Could you check a few things on this model? Use its own coordinates, in mm. A direction names the side the tool comes from. Round coordinates to 2 decimals unless told otherwise and drop trailing zeros. Order: outer loops, then holes, each group sorted by start corner. A loop starts at its lowest first (then second) coordinate and runs counter-clockwise, first axis right, second up.
```python
from build123d import *

# Parameters (mm, degrees)
F1_DEPTH  = 3
F3_DEPTH  = 10
F5_DEPTH  = 25
F6_W      = 4.4599839021
F6_H      = 15.0388356149
F6_W_2    = 4
F7_DEPTH  = 3
F8_R      = 1.5
F9_DEPTH  = 25
F11_DEPTH = 25


with BuildPart() as f1:
    # F0 (on Top) → F1 (new body)
    with BuildSketch(Plane.XY):
        with BuildLine():
            Line((1.9915475706, -41), (1.9915475706, -25.9236135266))
            ThreePointArc((1.9915475706, -25.9236135266), (0.0084775482, 25.9999986179), (-2.0084524294, -25.9223092883))
            Line((-2.0084524294, -25.9223092883), (-2.0084524294, -41))
            Line((-2.0084524294, -41), (1.9915475706, -41))
        make_face()
    extrude(amount=-F1_DEPTH)

    # F2 (on face) → F3 (join)
    with BuildSketch(Plane.XY):
        with BuildLine():
            Line((1.9915475706, 0), (-2.0153727382, 0))
            Line((-2.0153727382, 0), (-2.0153727382, -25.9217721756))
            ThreePointArc((-2.0153727382, -25.9217721756), (-2.0119126018, -25.9220409629), (-2.0084524294, -25.9223092883))
            Line((-2.0084524294, -25.9223092883), (-2.0084524294, -41))
            Line((-2.0084524294, -41), (1.9915475706, -41))
            Line((1.9915475706, -41), (1.9915475706, -25.9236135266))
            Line((1.9915475706, -25.9236135266), (1.9915475706, 0))
        make_face()
    extrude(amount=F3_DEPTH)

    # F4 (on face) → F5 (cut)
    with BuildSketch(Plane.YZ.offset(1.9915475706)):
        Polygon((-29.4827464968, 10), (0, 0), (0, 10), align=None)
    extrude(amount=-F5_DEPTH, mode=Mode.SUBTRACT)

    # F6 (on face) → F7 (cut)
    with BuildSketch(Plane(origin=(0, 0, -3), x_dir=(1, 0, 0), z_dir=(0, 0, -1))):
        with Locations((-0.0513555715, 33.4805821925)):
            Rectangle(F6_W, F6_H)
        with Locations((-0.0084524294, 33.4805821925)):
            Rectangle(F6_W_2, F6_H)
    extrude(amount=-F7_DEPTH, mode=Mode.SUBTRACT)

    # F8 (on face) → F9 (cut)
    with BuildSketch(Plane.YZ.offset(1.9915475706)):
        with Locations((-36, 5)):
            Circle(F8_R)
    extrude(amount=-F9_DEPTH, mode=Mode.SUBTRACT)

    # F10 (on face) → F11 (cut)
    with BuildSketch(Plane.YZ.offset(1.9915475706)):
        Polygon((-25.9236135266, -3), (-25.9236135266, 0), (-41, 1.5707125422), (-41, 0), (-25.9611643851, 0), (-25.9611643851, -3), align=None)
    extrude(amount=-F11_DEPTH, mode=Mode.SUBTRACT)


solid = f1.part
```
Q1. Imagine slicing it at C-C, the plane y = -36. Please give me the cut outline in (x, z), then the cut area to 3 significant figures.
Q2. For faces 4 (the flat face through (-2.015, -19, 2)), 5 (the flat face through (0, -41, 6)), 6 (the flat face through (0, -25.924, -2)), which set-ups out of +Z, -Z, +X, -X, +Y, -Y let a thin tool reach every point of the face, with its end or its side?
Q3. Imagine slicing it at D-D, the plane y = -19. Please give me the cut outline in (x, z), then the cut area to 3 significant figures.
Q4. We'd pull the mould along Z, two halves only. Please class faces 1 (the cylindrical face through (0, -37.2, 4.1)), 2 (the flat face through (0.02, -33.356, 0.774)), 3 (the flat face through (1.992, -25, 4)): released by +Z, released by -Z, zero draft, split by the parting line, or undercut.
Q5. For P1, Ø4.5, axis at y = -17.5, z = 3.5, coming from the -X side; P2, Ø6, axis at y = -9, z = 5, coming from the +X side; P3, Ø5, axis at x = -18.5, z = 1.5, coming from the -Y side; P4, Ø3, axis at x = 14.5, z = 3, coming from the +Y side, each with a flat end and sliding along its axis, tell me the tip position at first contact or that it passes through.
Q6. I need wall thicknesses on L1, parallel to Z at x = -1, y = -36; L2, parallel to Z at x = 23, y = -5.5; L3, parallel to X at y = -7, z = 2. Which ranges of each line are inside material? Lowest first, please.
Q7. Imagine slicing it at A-A, the plane x = 0. Please give me the cut outline in (y, z).
Filled in:
1. outline: (-2.01, 1.05) - (1.99, 1.05) - (1.99, 3.5) - (-2.01, 3.5) - close; (-2.01, 6.5) - (1.99, 6.5) - (1.99, 10) - (-2.01, 10) - close
1. area: 23.8 mm2
2. face 4: +Z, -X, +Y, -Y
2. face 5: +Z, -Z, +X, -X, -Y
2. face 6: -Z, +X, -X, -Y
3. outline: (-17.75, -3) - (17.75, -3) - (17.75, 0) - (1.99, 0) - (1.99, 6.44) - (-2.02, 6.44) - (-2.02, 0) - (-17.75, 0) - close
3. area: 132 mm2
4. face 1: undercut
4. face 2: released by -Z
4. face 3: zero draft
5. P1: stops at x = -2.02
5. P2: stops at x = 1.99
5. P3: stops at y = -20.09
5. P4: passes through
6. L1: z = 1.05 to 3.5, 6.5 to 10
6. L2: z = -3 to 0
6. L3: x = -2.02 to 1.99
7. outline: (-41, 1.57) - (-25.92, 0) - (-25.92, -3) - (26, -3) - (26, 0) - (0, 0) - (-29.48, 10) - (-41, 10) - close; hole circle Ø3 at (-36, 5)
